Geometry check sheet. Reference: the model listing, model coordinates, mm. Face numbers are marked on the shaded views. Coordinates: 2 decimals unless noted, no trailing zeros. Loops run counter-clockwise (first coordinate to the right, second up) from the corner with the lowest first, then second, coordinate; pieces in that order, holes last. Notation, with made-up numbers: (-3, -3.75) - (30, -3.75) arc R19 ccw to (30, 5.25) - close; hole circle Ø8 at (-2, 38). An arc over 180 degrees is marked (long way). Write item = value, one per line. Start each with the question number.
Autodesk Inventor part; units mm, degrees
ref_plane "YZ Plane" through (0, 0, 0) normal (1, 0, 0) x (0, 1, 0)
ref_plane "XZ Plane" through (0, 0, 0) normal (0, 1, 0) x (-1, 0, 0)
ref_plane "XY Plane" through (0, 0, 0) normal (0, 0, 1) x (1, 0, 0)
sketch "Sketch1" plane through (0, 0, 0) normal (1, 0, 0) x (0, 1, 0)
  line L0 (0, 0) -> (-59.252, 0)
  line L1 (-59.252, 0) -> (-59.252, -42.3)
  line L2 (-59.252, -42.3) -> (0, -42.3)
  line L3 (0, -42.3) -> (0, 0)
  line L4 (-59.252, -42.3) -> (-39.252, -42.3)
  line L5 (-39.252, -42.3) -> (-39.252, 0)
  line L6 (-39.252, 0) -> (-59.252, 0)
  line L7 (-59.252, 0) -> (-59.252, -42.3)
  line L8 (-59.252, 0) -> (-49.252, 0)
  line L9 (-49.252, 0) -> (-49.252, -21.15)
  line L10 (-49.252, -21.15) -> (-49.252, -31.725)
  circle A0 centre (-49.252, -31.725) radius 3
  line L11 (-49.252, -21.15) -> (-49.252, -10.575)
  circle A1 centre (-49.252, -10.575) radius 3
  circle A2 centre (0, -21.15) radius 10
  line L12 (0, 0) -> (21.15, 0)
  line L13 (21.15, 0) -> (21.15, -42.3)
  line L14 (21.15, -42.3) -> (0, -42.3)
  line L15 (0, -42.3) -> (0, 0)
  line L16 (0, -21.15) -> (0, -36.65)
  line L17 (0, -36.65) -> (15.5, -36.65)
  circle A3 centre (15.5, -36.65) radius 2
  circle A4 centre (-15.5, -36.65) radius 2
  circle A5 centre (15.5, -5.65) radius 2
  circle A6 centre (-15.5, -5.65) radius 2
  dimension "d1" = 59.252
  dimension "d2" = 42.3
  dimension "d3" = 20
  dimension "d4" = 10
  dimension "d5" = 21.15
  dimension "d6" = 10.575
  dimension "d7" = 6
  dimension "d8" = 10.575
  dimension "d9" = 6
  dimension "d10" = 20
  dimension "d11" = 21.15
  dimension "d12" = 15.5
  dimension "d13" = 15.5
  dimension "d14" = 4
  dimension "d17" = 31
  dimension "d20" = 31
extrude "Extrusion1" add sketch "Sketch1" along normal blind 2 contours L3 A2 L2 L5 L0 | L12 L13 L14 L3 A2 | L5 L2 L1 L0
properties part number "az_rot_mot_holder.iam" material "Aluminum 6061"
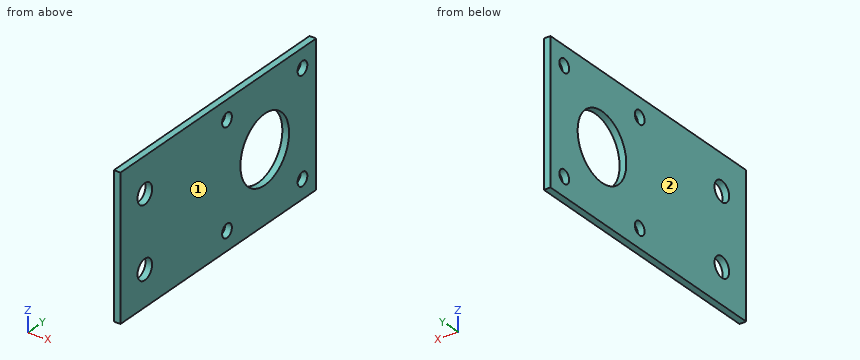
(1) Sectioned sample at B-B on z = -36.65. Enter the section's corners in (x, y), plus the area to 3 significant figures.
(2) Scan lines: line 1 (Z direction, x = 1.5, y = -15.5); line 2 (Z direction, x = 1.3, y = 14.5); line 3 (Y direction, x = 0.6, z = -30). Record each from-to range of solid material in increasing order.
(3) Sectioned sample at C-C on y = 0. Enter the section's corners in (x, z), plus the area to 3 significant figures.
(4) Depth check by flat-ended pin: pin 1 (3.5 mm diameter, centred on y = -15.5, z = -5.65, fed in from +X). Enter the tip coordinate at first touch or a pass-through.
(5) Draft check along X on the marked faces 1 and 2. Enter one of: pulls with the +X half, pulls with the -X half, needs draft (parallel to the pull), parting line crosses it, or undercut.
(6) Sectioned sample at D-D on x = 0.3. Enter the section's corners in (y, z) (3 decimals).
(7) Sectioned sample at A-A on y = 15.5. Enter the section's corners in (x, z).
Working result:
q1.outline = (0, -59.25) - (2, -59.25) - (2, -17.5) - (0, -17.5) - close; (0, -13.5) - (2, -13.5) - (2, 13.5) - (0, 13.5) - close; (0, 17.5) - (2, 17.5) - (2, 21.15) - (0, 21.15) - close
q1.area = 145 mm2
q2.line_1 = -42.3 to -38.65, -34.65 to -7.65, -3.65 to 0
q2.line_2 = -42.3 to -38.38, -34.92 to -7.38, -3.92 to 0
q2.line_3 = -59.25 to -51.71, -46.8 to -4.66, 4.66 to 21.15
q3.outline = (0, -42.3) - (2, -42.3) - (2, -31.15) - (0, -31.15) - close; (0, -11.15) - (2, -11.15) - (2, 0) - (0, 0) - close
q3.area = 44.6 mm2
q4.pin_1 = through
q5.face_1 = pulls with the +X half
q5.face_2 = pulls with the -X half
q6.outline = (-59.252, -42.3) - (21.15, -42.3) - (21.15, 0) - (-59.252, 0) - close; hole circle Ø6 at (-49.252, -31.725); hole circle Ø6 at (-49.252, -10.575); hole circle Ø4 at (-15.5, -36.65); hole circle Ø4 at (-15.5, -5.65); hole circle Ø20 at (0, -21.15); hole circle Ø4 at (15.5, -36.65); hole circle Ø4 at (15.5, -5.65)
q7.outline = (0, -42.3) - (2, -42.3) - (2, -38.65) - (0, -38.65) - close; (0, -34.65) - (2, -34.65) - (2, -7.65) - (0, -7.65) - close; (0, -3.65) - (2, -3.65) - (2, 0) - (0, 0) - close
